```python
from build123d import *

# Parameters (mm, degrees)
SKETCH_2_R          = 13.25
SKETCH_2_R_2        = 1.6
EXTRUDE_1_DEPTH     = 3
FILLET_3_R          = 5
SKETCH_4_R          = 1.5
SKETCH_4_R_2        = 1.1
SKETCH_4_W          = 5
SKETCH_4_H          = 20
CUT_EXTRUDE_1_DEPTH = 10


with BuildPart() as part:
    # ｽｹｯﾁ2 → ﾎﾞｽ - 押し出し1 (new body)
    with BuildSketch(Plane.XY):
        with BuildLine():
            Line((-60, -22.5), (-40, -22.5))
            Line((-40, -22.5), (0, -22.5))
            ThreePointArc((0, -22.5), (19.65247344, -10.9558335), (19.138597944, 11.830641096))
            Line((19.138597944, 11.830641096), (-40, 107.5))
            Line((-40, 107.5), (-60, 107.5))
            Line((-60, 107.5), (-60, -22.5))
        make_face()
        Circle(SKETCH_2_R, mode=Mode.SUBTRACT)
        with Locations((0, 17.5)):
            Circle(SKETCH_2_R_2, mode=Mode.SUBTRACT)
        with Locations((17.5, 0)):
            Circle(SKETCH_2_R_2, mode=Mode.SUBTRACT)
        with Locations((0, -17.5)):
            Circle(SKETCH_2_R_2, mode=Mode.SUBTRACT)
        with Locations((-17.5, 0)):
            Circle(SKETCH_2_R_2, mode=Mode.SUBTRACT)
    extrude(amount=EXTRUDE_1_DEPTH)

    # ﾌｨﾚｯﾄ3
    fillet_3_edges = [part.edges().sort_by_distance(p)[0] for p in [
        (-40, 107.5, 1.5),
    ]]
    fillet(fillet_3_edges, radius=FILLET_3_R)

    # ｽｹｯﾁ4 → ｶｯﾄ - 押し出し1 (cut)
    with BuildSketch(Plane.XY.offset(3)):
        with Locations((-57.5, -7.5)):
            Circle(SKETCH_4_R)
        with Locations((-57.5, 42.5)):
            Circle(SKETCH_4_R)
        with Locations((-57.5, 92.5)):
            Circle(SKETCH_4_R)
        with Locations((-55.66, 26.84)):
            Circle(SKETCH_4_R_2)
        with Locations((-55.66, 8.16)):
            Circle(SKETCH_4_R_2)
        with Locations((-55.66, 58.16)):
            Circle(SKETCH_4_R_2)
        with Locations((-55.66, 76.84)):
            Circle(SKETCH_4_R_2)
        with Locations((-57.5, 67.5)):
            Rectangle(SKETCH_4_W, SKETCH_4_H)
        with Locations((-57.5, 17.5)):
            Rectangle(SKETCH_4_W, SKETCH_4_H)
    extrude(amount=-CUT_EXTRUDE_1_DEPTH, mode=Mode.SUBTRACT)


solid = part.part
```
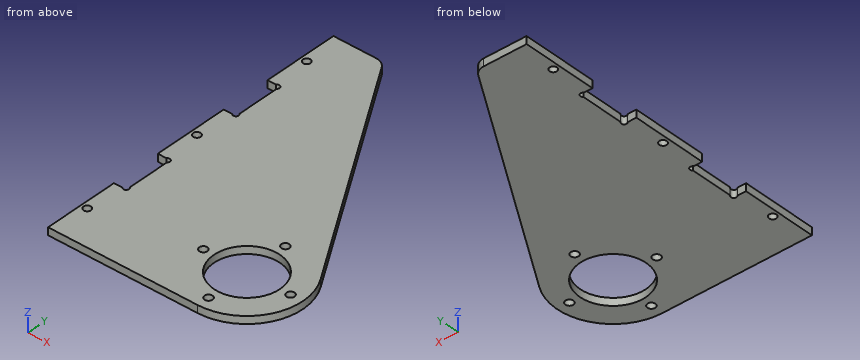
Could you check a few things on this model? Use its own coordinates, in mm. Round coordinates to 2 decimals unless told otherwise and drop trailing zeros. Loops run counter-clockwise (first coordinate to the right, second up) from the corner with the lowest first, then second, coordinate; pieces in that order, holes last. Notation, with made-up numbers: M -13.75,22.5 L 36.25,22.5 A10 cw 36.25,40.5 Z; hole C 79,26.5 d4. An arc over 180 degrees is marked long. Write item = value, one per line.
1. I want a section at A-A, the plane z = 1.95. Count the separate pieces of the cut face and the enclosed holes in it, and give its area (3 significant figures).
Results below:
separate_pieces = 1
enclosed_holes = 8
area = 6,640 mm²
2. Will these pins go through, and if not, where does the flat tip stop? P1, Ø3, axis at x = -55.66, y = 8.16, coming from the -Z side; P2, Ø0.9, axis at y = 17.5, z = 1, coming from the -X side.
Results below:
P1 = 0
P2 = -55
3. I need wall thicknesses on probe 1 along Y at (x, z) = (-55.66, 1.6); probe 2 along Y at (x, z) = (-57.5, 2.05); probe 3 along Y at (x, z) = (0, 2.4). Which ranges of each line are inside material? Lowest first, please.
Results below:
probe_1 = -22.5 to 7.06, 27.94 to 57.06, 77.94 to 107.5
probe_2 = -22.5 to -9, -6 to 7.5, 27.5 to 41, 44 to 57.5, 77.5 to 91, 94 to 107.5
probe_3 = -22.5 to -19.1, -15.9 to -13.25, 13.25 to 15.9, 19.1 to 42.79
4. I want a section at C-C, the plane x = 6. Write out the boundary of the cut face in (y, z), and give its area (3 significant figures).
Results below:
outline = M -21.69,0 L -11.81,0 L -11.81,3 L -21.69,3 Z; M 11.81,0 L 33.09,0 L 33.09,3 L 11.81,3 Z
area = 93.4 mm²
5. I want a section at D-D, the plane y = 42.5. Write out the boundary of the cut face in (x, z), and give its area (3 significant figures).
Results below:
outline = M -60,0 L -59,0 L -59,3 L -60,3 Z; M -56,0 L 0.18,0 L 0.18,3 L -56,3 Z
area = 172 mm²
6. I want a section at B-B, the plane y = 0. Write out the boundary of the cut face in (x, z).
Results below:
outline = M -60,0 L -19.1,0 L -19.1,3 L -60,3 Z; M -15.9,0 L -13.25,0 L -13.25,3 L -15.9,3 Z; M 13.25,0 L 15.9,0 L 15.9,3 L 13.25,3 Z; M 19.1,0 L 22.5,0 L 22.5,3 L 19.1,3 Z
